Answer from the drawing. Dimensions are ordinates in mm from the lowest x, y and z of the part. A direction names the side the tool comes from. Give positions to 0.01 mm unless a question says otherwise; leave off trailing zeros. Write each loop counter-clockwise with the first axis right and the second up, starting at its lowest first coordinate (ties: lowest second). Pieces come first, ordered by that corner, then holes. Notation, with made-up numbers: (41, 24.5) -> (88, 24.5) arc R20 ccw to (88, 62.5) -> close; hole circle Ø10 at (19.25, 33). An arc over 180 degrees is marked (long way). Write item = value, one per line.
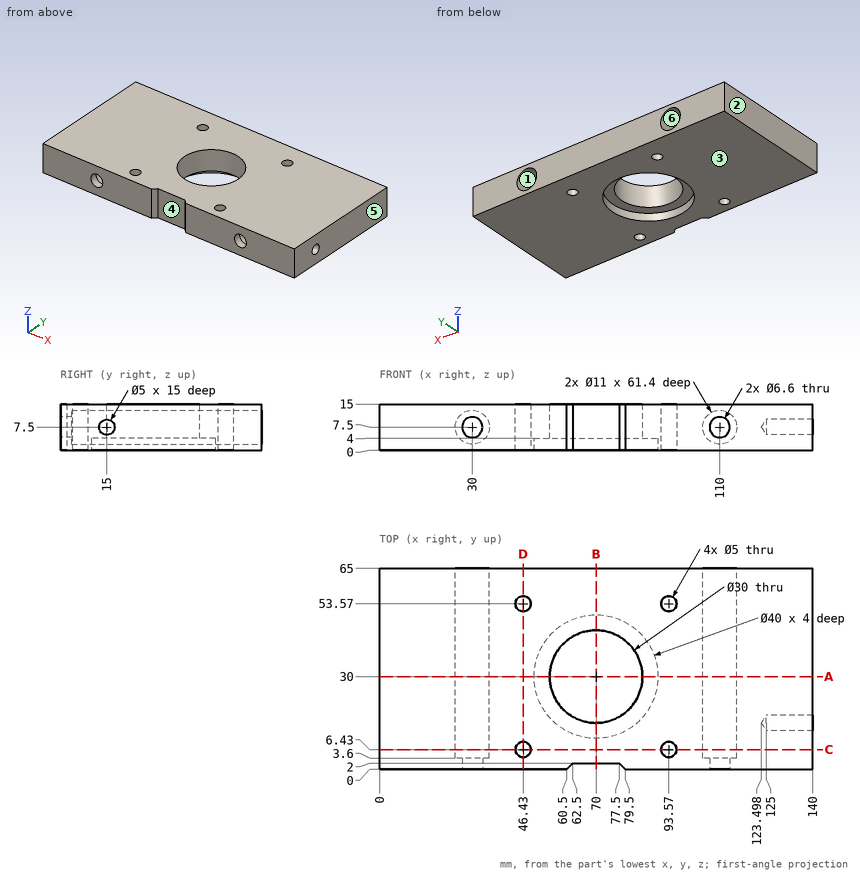
(1) The part is cut by section D-D on x = 46.43. Determine the outline of the cut face in (y, z), plus the area to 3 significant figures.
Checks:
outline = (0, 0) -> (3.93, 0) -> (3.93, 15) -> (0, 15) -> close; (8.93, 0) -> (51.07, 0) -> (51.07, 15) -> (8.93, 15) -> close; (56.07, 0) -> (65, 0) -> (65, 15) -> (56.07, 15) -> close
area = 825 mm²
(2) The part is cut by section C-C on y = 6.43. Determine the outline of the cut face in (x, z), plus the area to 3 significant figures.
Checks:
outline = (0, 0) -> (43.93, 0) -> (43.93, 15) -> (0, 15) -> close; (48.93, 0) -> (91.07, 0) -> (91.07, 15) -> (48.93, 15) -> close; (96.07, 0) -> (140, 0) -> (140, 15) -> (96.07, 15) -> close; hole circle Ø11 at (30, 7.5); hole circle Ø11 at (110, 7.5)
area = 1,760 mm²
(3) The part is cut by section B-B on x = 70. Determine the outline of the cut face in (y, z).
Checks:
outline = (2, 0) -> (10, 0) -> (10, 4) -> (15, 4) -> (15, 15) -> (2, 15) -> close; (45, 4) -> (50, 4) -> (50, 0) -> (65, 0) -> (65, 15) -> (45, 15) -> close
(4) For a pull along X with two mould halves and no side action, classify the marked faces 1, 2 and 3 as released by +X, released by -X, zero draft, split by the parting line, or undercut.
Checks:
face_1 = undercut
face_2 = released by -X
face_3 = zero draft
(5) The part is cut by section A-A on y = 30. Determine the outline of the cut face in (x, z), plus the area to 3 significant figures.
Checks:
outline = (0, 0) -> (50, 0) -> (50, 4) -> (55, 4) -> (55, 15) -> (0, 15) -> close; (85, 4) -> (90, 4) -> (90, 0) -> (140, 0) -> (140, 15) -> (85, 15) -> close; hole circle Ø11 at (30, 7.5); hole circle Ø11 at (110, 7.5)
area = 1,420 mm²
(6) Consider L1, parallel to X at y = 58, z = 7; L2, parallel to Y at x = 93.57, z = 3.75; L3, parallel to X at y = 53.57, z = 8. Determine where each line is inside the solid, lowest interval first.
Checks:
L1 = 0 to 24.52, 35.48 to 104.52, 115.48 to 140
L2 = 0 to 3.93, 8.93 to 51.07, 56.07 to 65
L3 = 0 to 24.52, 35.48 to 43.93, 48.93 to 91.07, 96.07 to 104.52, 115.48 to 140
(7) Given P1, Ø5.5, axis at x = 112, z = 9, coming from the +Y side; P2, Ø7.5, axis at x = 67.5, z = 8, coming from the -Y side, each flat-ended and moving along its own axis, determine where each tip first touches the part or whether it passes through.
Checks:
P1 = 3.6
P2 = 2
(8) A tool of negligible diameter and unlimited length cuts with its end or side. For the marked faces 4, 5 and 6, from which of +Z, -Z, +X, -X, +Y, -Y can it reach the whole face along a straight path? Write none if from no direction.
Checks:
face_4 = +Z, -Z, -Y
face_5 = +Z, -Z, +X, +Y, -Y
face_6 = +Y
